CAD build for the part. Positions are in the model's coordinates, mm. Face numbers are marked on the shaded views. A direction names the side the tool comes from. Round coordinates to 2 decimals unless told otherwise and drop trailing zeros. Write each loop counter-clockwise with the first axis right and the second up, starting at its lowest first coordinate (ties: lowest second). Pieces come first, ordered by that corner, then holes. Notation, with made-up numbers: (67.25, 42) - (72.25, 42) arc R28 ccw to (72.25, 74) - close; hole circle Ø2 at (-31.5, 27.25). An arc over 180 degrees is marked (long way). Put each result on its own line as item: value. Start each with the question number.
Item 1: 3-axis set-ups, long thin cutter, end or side, ignore diameter. For the marked faces 4 and 5: which of +Z, -Z, +X, -X, +Y, -Y reach the whole face in a straight line?
Item 2: Cut at D-D (z = -14.9). Give the cut face in (x, y), and give its area (3 significant figures).
Item 3: Mould opens along X. For the marked faces 1, 2 and 3 say: released by +X, released by -X, zero draft, split by the parting line, or undercut.
Item 4: Pin check, flat tips, straight feed: pin 1 Ø4 at (x, y) = (-8, 5.5) entering from -Z; pin 2 Ø2.5 at (x, z) = (8, -7.9) entering from -Y; pin 3 Ø10 at (x, z) = (-5.5, -17) entering from +Y. Stop position of each tip, or through.
Item 5: Cut at A-A (x = 0). Give the cut face in (y, z).
Item 6: Cut at C-C (x = -8.5). Give the cut face in (y, z), and give its area (3 significant figures).
Item 7: Cut at B-B (z = -21.9). Give the cut face in (x, y).
Item 8: Drill centre lines: line 1 (X direction, y = -16, z = -21.9); line 2 (Y direction, x = -3.25, z = -28); line 3 (Z direction, x = 0, y = 10.5). Where is each one in solid material? Low to high. Write a range as from..to.
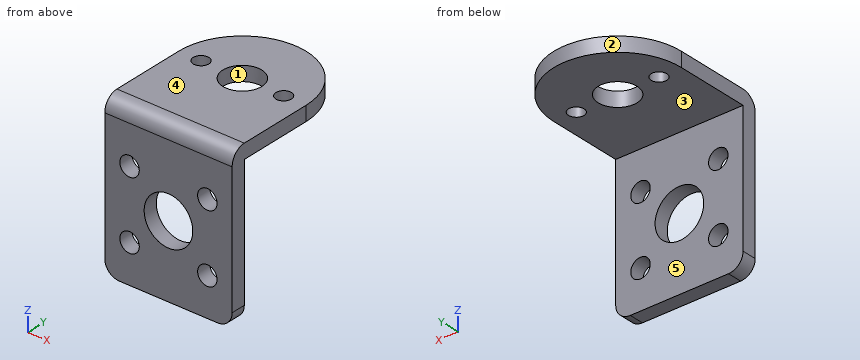
```python
from build123d import *

# Parameters (mm, degrees)
SKETCH1_R            = 4
SKETCH1_R_2          = 1.6
JGA25_SCREWS_DEPTH   = 3
SKETCH2_W            = 26.2
SKETCH2_H            = 29.8
SKETCH2_R            = 5
SKETCH2_R_2          = 2
BRACKET_SCREWS_DEPTH = 3
L_SHAPE_FILLET_R     = 3
CORNER_FILLETS_R     = 3


with BuildPart() as part:
    # Sketch1 → JGA25-Screws (new body)
    with BuildSketch(Plane.XY):
        with BuildLine():
            Line((-13.1, 0), (-13.1, -18.25))
            Line((-13.1, -18.25), (13.1, -18.25))
            Line((13.1, -18.25), (13.1, 0))
            ThreePointArc((13.1, 0), (0, 13.1), (-13.1, 0))
        make_face()
        Circle(SKETCH1_R, mode=Mode.SUBTRACT)
        with Locations((-8.5, 0)):
            Circle(SKETCH1_R_2, mode=Mode.SUBTRACT)
        with Locations((8.5, 0)):
            Circle(SKETCH1_R_2, mode=Mode.SUBTRACT)
    extrude(amount=JGA25_SCREWS_DEPTH)

    # Sketch2 → Bracket-Screws (add)
    with BuildSketch(Plane.XZ.offset(18.25)):
        with Locations((0, -14.9)):
            Rectangle(SKETCH2_W, SKETCH2_H)
        with Locations(Location((0, -14.9, 0), (0, 0, 270))):
            Circle(SKETCH2_R, mode=Mode.SUBTRACT)
        with Locations(Location((8, -21.9, 0), (0, 0, 270))):
            Circle(SKETCH2_R_2, mode=Mode.SUBTRACT)
        with Locations(Location((-8, -21.9, 0), (0, 0, 270))):
            Circle(SKETCH2_R_2, mode=Mode.SUBTRACT)
        with Locations(Location((8, -7.9, 0), (0, 0, 270))):
            Circle(SKETCH2_R_2, mode=Mode.SUBTRACT)
        with Locations(Location((-8, -7.9, 0), (0, 0, 270))):
            Circle(SKETCH2_R_2, mode=Mode.SUBTRACT)
    extrude(amount=-BRACKET_SCREWS_DEPTH)

    # L-Shape-Fillet
    l_shape_fillet_edges = [part.edges().sort_by_distance(p)[0] for p in [
        (0, -18.25, 3),
    ]]
    fillet(l_shape_fillet_edges, radius=L_SHAPE_FILLET_R)

    # Corner-Fillets
    corner_fillets_edges = [part.edges().sort_by_distance(p)[0] for p in [
        (-13.1, -16.75, -29.8),
        (13.1, -16.75, -29.8),
    ]]
    fillet(corner_fillets_edges, radius=CORNER_FILLETS_R)


solid = part.part
```
Output values:
1. face 4: +Z, +X, -X, +Y, -Y
1. face 5: -Z, +X, -X, +Y
2. outline: (-13.1, -18.25) - (-5, -18.25) - (-5, -15.25) - (-13.1, -15.25) - close; (5, -18.25) - (13.1, -18.25) - (13.1, -15.25) - (5, -15.25) - close
2. area: 48.6 mm2
3. face 1: undercut
3. face 2: split by the parting line
3. face 3: zero draft
4. pin 1: z = 0
4. pin 2: through
4. pin 3: y = -15.25
5. outline: (-18.25, -29.8) - (-15.25, -29.8) - (-15.25, -19.9) - (-18.25, -19.9) - close; (-18.25, -9.9) - (-15.25, -9.9) - (-15.25, 0) - (-4, 0) - (-4, 3) - (-15.25, 3) arc R3 ccw to (-18.25, 0) - close; (4, 0) - (13.1, 0) - (13.1, 3) - (4, 3) - close
6. outline: (-18.25, -29.8) - (-15.25, -29.8) - (-15.25, -23.84) - (-18.25, -23.84) - close; (-18.25, -19.96) - (-15.25, -19.96) - (-15.25, -9.84) - (-18.25, -9.84) - close; (-18.25, -5.96) - (-15.25, -5.96) - (-15.25, 0) - (-1.6, 0) - (-1.6, 3) - (-15.25, 3) arc R3 ccw to (-18.25, 0) - close; (1.6, 0) - (9.97, 0) - (9.97, 3) - (1.6, 3) - close
6. area: 139 mm2
7. outline: (-13.1, -18.25) - (-10, -18.25) - (-10, -15.25) - (-13.1, -15.25) - close; (-6, -18.25) - (6, -18.25) - (6, -15.25) - (-6, -15.25) - close; (10, -18.25) - (13.1, -18.25) - (13.1, -15.25) - (10, -15.25) - close
8. line 1: -13.1..-10, -6..6, 10..13.1
8. line 2: -18.25..-15.25
8. line 3: 0..3
